from build123d import *
from build123d.topology import SkipClean

# Parameters (mm, degrees)
SCHIZZO1_R                  = 11
SCHIZZO1_R_2                = 9.25
TUBO_DEPTH                  = 210
INGRESSOCAVI_DEPTH          = 27
SCHIZZO4_R                  = 11
SCHIZZO4_R_2                = 6.5
FONDOCORSA_DEPTH            = 3
SCHIZZO5_R                  = 11
TAPPO_DEPTH                 = 2
BASEINFERIORE_DEPTH         = 239
SCHIZZO7_R                  = 13.5
TAGLIOANELLO_DEPTH          = 15
SUPPORTOANELLO_DEPTH        = 15
FACILITAZIONECAVI_DEPTH     = 3
RACCORDOFACILITAZIONECAVI_R = 8


with BuildPart() as part:
    # Schizzo1 → Tubo (new body)
    with BuildSketch(Plane.XY):
        Circle(SCHIZZO1_R)
        Circle(SCHIZZO1_R_2, mode=Mode.SUBTRACT)
    extrude(amount=TUBO_DEPTH)

    # Schizzo2 → IngressoCavi (add)
    with BuildSketch(Plane.XY.offset(210)):
        with BuildLine():
            Line((0, -9.25), (0, -11))
            ThreePointArc((0, -11), (-7.778174593, 7.778174593), (11, 0))
            Line((11, 0), (9.25, 0))
            ThreePointArc((9.25, 0), (-6.540737726, 6.540737726), (0, -9.25))
        make_face()
    extrude(amount=INGRESSOCAVI_DEPTH)

    # Schizzo4 → FondoCorsa (add)
    with SkipClean():  # the faces are left unmerged after this step: merging them gives an invalid solid
        with BuildSketch(Plane.XY.offset(210)):
            Circle(SCHIZZO4_R)
            Circle(SCHIZZO4_R_2, mode=Mode.SUBTRACT)
        extrude(amount=FONDOCORSA_DEPTH)

    # Schizzo5 → Tappo (add)
    with SkipClean():  # the faces are left unmerged after this step: merging them gives an invalid solid
        with BuildSketch(Plane.XY.offset(237)):
            Circle(SCHIZZO5_R)
        extrude(amount=TAPPO_DEPTH)
    add(part.part.scale(1), mode=Mode.REPLACE)  # the faces are merged on a copy

    # Schizzo6 → BaseInferiore (add)
    with BuildSketch(Plane.XY):
        Polygon((-2.5, 11), (-2.5, 15), (2.5, 15), (2.5, 11), (2.5, 10.712142643), (-2.5, 10.712142643), align=None)
    extrude(amount=BASEINFERIORE_DEPTH)

    # Schizzo7 → TaglioAnello (cut)
    with BuildSketch(Plane.XY.offset(73.5)):
        Circle(SCHIZZO7_R)
    extrude(amount=-TAGLIOANELLO_DEPTH, mode=Mode.SUBTRACT)

    # Schizzo8 → SupportoAnello (add)
    with BuildSketch(Plane.XY.offset(73.5)):
        with BuildLine():
            Line((0, 15), (0, 13.5))
            ThreePointArc((0, 13.5), (-9.545941546, 9.545941546), (-13.5, 0))
            Line((-13.5, 0), (-15, 0))
            ThreePointArc((-15, 0), (-10.606601718, 10.606601718), (0, 15))
        make_face()
    extrude(amount=-SUPPORTOANELLO_DEPTH)

    # Schizzo9 → FacilitazioneCavi (cut)
    with BuildSketch(Plane(origin=(0, 0, 210), x_dir=(-1, 0, 0), z_dir=(0, 0, -1))):
        with BuildLine():
            Line((0, -9.25), (0, 0))
            Line((0, 0), (-9.25, 0))
            ThreePointArc((-9.25, 0), (-6.540737726, -6.540737726), (0, -9.25))
        make_face()
    extrude(amount=-FACILITAZIONECAVI_DEPTH, mode=Mode.SUBTRACT)

    # RaccordoFacilitazioneCavi
    # the kernel refuses this fillet: 8 mm, written as the material it takes off along each edge
    with BuildSketch(Plane(origin=(6.5, 0, 201.530207244), x_dir=(1, 0, 0), z_dir=(0, 0, 1)), Plane(origin=(0, -6.5, 221.469792756), x_dir=(0, -1, 0), z_dir=(0, 0, -1))) as raccordofacilitazionecavi_piece_1:
        with BuildLine():
            CenterArc((6.030405405, 7.296501927), RACCORDOFACILITAZIONECAVI_R, 210.212403153, 35.579578639)
            Line((-0.882921715, 3.270845692), (-1.021188257, 3.190332567))
            ThreePointArc((-1.021188257, 3.190332567), (-0.379082322, 1.65226111), (-0.16, 0))
            Line((-0.16, 0), (0, -0.16))
            ThreePointArc((0, -0.16), (1.375, -0.16), (2.684391892, -0.145930039))
            Line((2.684391892, -0.145930039), (2.75, 0))
        make_face()
    extrude(amount=19.939585512, mode=Mode.SUBTRACT)


solid = part.part
Input: part model. Units: mm. Frame: model coordinates. A direction names the side the tool comes from. Give positions to 0.01 mm unless a question says otherwise; leave off trailing zeros. Loops run counter-clockwise (first coordinate to the right, second up) from the corner with the lowest first, then second, coordinate; pieces in that order, holes last. Notation, with made-up numbers: (48.5, -33.75) -> (106.5, -33.75) arc R14 cw to (106.5, -9.75) -> close; hole circle Ø11 at (-24, 48.25). An arc over 180 degrees is marked (long way). Answer as a JSON object with one key per item and string values. Group by question number.
Item 1: Line query: probe 1 along Y at (x, z) = (0, 212.25); probe 2 along X at (y, z) = (0, 211.7); probe 3 along X at (y, z) = (0, 109). Output: solid intervals per line, ascending.
Item 2: Cut plane A-A, the plane z = 120.5. Return the cut outline in (x, y).
Item 3: Pin query (flat end, axial travel): P1, Ø1.5, axis at y = 8, z = 119, coming from the +X side; P2, Ø6, axis at x = -12, z = 151, coming from the +Y side; P3, Ø9, axis at x = -2.5, y = -2.5, coming from the -Z side. Return the tip coordinate at first contact, or that it passes through.
Item 4: Reachability of faces 5 (the flat face through (-11, 9, 73.5)), 6 (the flat face through (2.5, 13, 118)), 7 (the cylindrical face through (-2.01, -9.03, 28.84)), 8 (the flat face through (1, -1, 237)) from +Z, -Z, +X, -X, +Y, -Y: full face, straight path, thin tool, end or side. Return the list, or none.
Item 5: Pull-direction query (Z, two-part tool) for faces 1 (the cylindrical face through (-4.48, 4.71, 211.48)), 2 (the flat face through (-0.9, 9.5, 58.5)), 3 (the flat face through (-4, 6, 213)), 4 (the flat face through (-11, 9, 58.5)); classes: released by +Z, released by -Z, zero draft, split by the parting line, or undercut.
Checks:
{
 "1": {"probe 1": "y = -11 to -9.25, 6.5 to 15", "probe 2": "x = -11 to -6.5, 9.25 to 11", "probe 3": "x = -11 to -9.25, 9.25 to 11"},
 "2": {"outline": "(-2.5, 10.71) arc R11 ccw (long way) to (2.5, 10.71) -> (2.5, 15) -> (-2.5, 15) -> close; hole circle Ø18.5 at (0, 0)"},
 "3": {"P1": "stops at x = 8.27", "P2": "stops at y = 6.32", "P3": "stops at z = 210"},
 "4": {"face 5": "+Z, -X, +Y", "face 6": "+Z, -Z, +X, +Y", "face 7": "-Z", "face 8": "none"},
 "5": {"face 1": "zero draft", "face 2": "undercut", "face 3": "undercut", "face 4": "released by -Z"}
}
